The model under review builds one solid part; all positions refer to its coordinate system, in mm. Give positions to 0.01 mm unless a question says otherwise; leave off trailing zeros. Write each loop counter-clockwise with the first axis right and the second up, starting at its lowest first coordinate (ties: lowest second). Pieces come first, ordered by that corner, then holes.
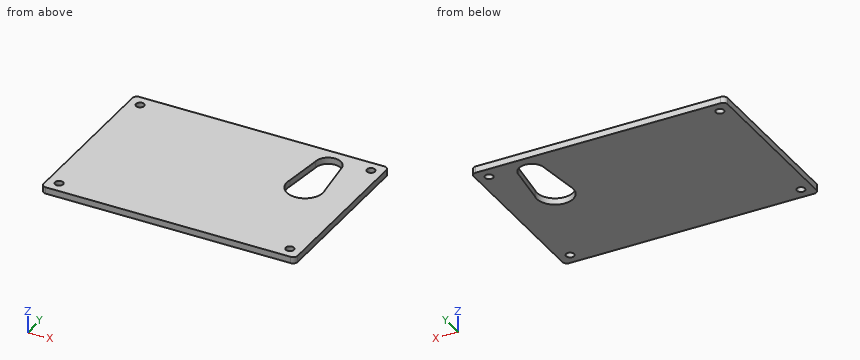
from build123d import *

# Parameters (mm, degrees)
SKETCH1_R           = 1.25
BOSS_EXTRUDE1_DEPTH = 2


with BuildPart() as part:
    # Sketch1 → Boss-Extrude1 (new body)
    with BuildSketch(Plane.XY):
        with BuildLine():
            ThreePointArc((48.610141298, 25.924362859), (48.207413123, 26.896634683), (47.235141298, 27.299362859))
            Line((47.235141298, 27.299362859), (-28.164858702, 27.299362859))
            ThreePointArc((-28.164858702, 27.299362859), (-29.137130526, 26.896634683), (-29.539858702, 25.924362859))
            Line((-29.539858702, 25.924362859), (-29.539858702, -24.475637141))
            ThreePointArc((-29.539858702, -24.475637141), (-29.137130526, -25.447908965), (-28.164858702, -25.850637141))
            Line((-28.164858702, -25.850637141), (47.235141298, -25.850637141))
            ThreePointArc((47.235141298, -25.850637141), (48.207413123, -25.447908965), (48.610141298, -24.475637141))
            Line((48.610141298, -24.475637141), (48.610141298, 25.924362859))
        make_face()
        with Locations((-25.964858702, -22.275637141)):
            Circle(SKETCH1_R, mode=Mode.SUBTRACT)
        with Locations((45.035141298, -22.275637141)):
            Circle(SKETCH1_R, mode=Mode.SUBTRACT)
        with Locations((-25.964858702, 23.724362859)):
            Circle(SKETCH1_R, mode=Mode.SUBTRACT)
        with BuildLine():
            ThreePointArc((29.638141298, 20.602682845), (33.575141298, 24.539682845), (37.512141298, 20.602682845))
            Line((37.512141298, 20.602682845), (38.989636745, 8.837022391))
            ThreePointArc((38.989636745, 8.837022391), (33.575141298, 1.867362859), (28.160645852, 8.837022391))
            Line((28.160645852, 8.837022391), (29.638141298, 20.602682845))
        make_face(mode=Mode.SUBTRACT)
        with Locations((45.035141298, 23.724362859)):
            Circle(SKETCH1_R, mode=Mode.SUBTRACT)
    extrude(amount=BOSS_EXTRUDE1_DEPTH)


solid = part.part
1) Consider section A-A, the plane y = 15. Give the boundary of the cut face in (x, z), then the cut area to 3 significant figures.
2) Consider section C-C, the plane y = 6.5. Give the boundary of the cut face in (x, z).
3) Consider section B-B, the plane z = 1.25. Give the boundary of the cut face in (x, y) (3 decimals), then the cut area to 3 significant figures.
4) To check wall thickness, follow probe 1 along Y at (x, z) = (45, 0.2); probe 2 along Y at (x, z) = (44.5, 0.9); probe 3 along Y at (x, z) = (37, 0.95). State the ranges of each line that lie inside material, in increasing order.
5) Insertion check: pin 1 (3 mm diameter, centred on x = -25.96, y = 23.72, fed in from -Z); pin 2 (1.5 mm diameter, centred on x = 45.04, y = -22.28, fed in from -Z). Each pin has a flat end and moves straight along its axis. Give the tip position at first contact, or say it passes through.
Answer block:
1. outline: (-29.54, 0) - (28.93, 0) - (28.93, 2) - (-29.54, 2) - close; (38.22, 0) - (48.61, 0) - (48.61, 2) - (38.22, 2) - close
1. area: 138 mm2
2. outline: (-29.54, 0) - (28.07, 0) - (28.07, 2) - (-29.54, 2) - close; (39.08, 0) - (48.61, 0) - (48.61, 2) - (39.08, 2) - close
3. outline: (-29.54, -24.476) arc R1.375 ccw to (-28.165, -25.851) - (47.235, -25.851) arc R1.375 ccw to (48.61, -24.476) - (48.61, 25.924) arc R1.375 ccw to (47.235, 27.299) - (-28.165, 27.299) arc R1.375 ccw to (-29.54, 25.924) - close; hole circle Ø2.5 at (-25.965, -22.276); hole circle Ø2.5 at (-25.965, 23.724); hole (28.161, 8.837) arc R5.588 ccw (long way) to (38.99, 8.837) - (37.512, 20.603) arc R3.937 ccw to (29.638, 20.603) - close; hole circle Ø2.5 at (45.035, -22.276); hole circle Ø2.5 at (45.035, 23.724)
3. area: 3,930 mm2
4. probe 1: y = -25.85 to -23.53, -21.03 to 22.47, 24.97 to 27.3
4. probe 2: y = -25.85 to -23.41, -21.15 to 22.59, 24.85 to 27.3
4. probe 3: y = -25.85 to 3.04, 22.54 to 27.3
5. pin 1: stops at z = 0
5. pin 2: passes through
